from build123d import *

# Parameters (mm, degrees)
SKETCH1_W                   = 127
SKETCH1_H                   = 127
BOSS_EXTRUDE1_DEPTH         = 3.175
F_16_0_177_DIAMETER_HOLE1_D = 4.4958
F_16_0_177_DIAMETER_HOLE2_D = 4.4958
SKETCH12_W                  = 6.35
SKETCH12_H                  = 19.05
CUT_EXTRUDE1_DEPTH          = 131.218638569
FILLET1_R                   = 2.54


with BuildPart() as part:
    # Sketch1 → Boss-Extrude1 (new body)
    with BuildSketch(Plane(origin=(0, 0, 0), x_dir=(1, 0, 0), z_dir=(0, 1, 0))):
        with Locations((-41.826357018, 13.006024096)):
            Rectangle(SKETCH1_W, SKETCH1_H)
    extrude(amount=BOSS_EXTRUDE1_DEPTH)

    # #16 (0.177) Diameter Hole1 (through all)
    with Locations(Plane(origin=(0, 0, 0), x_dir=(-1, 0, 0), z_dir=(0, -1, 0))):
        with Locations((3.726357018, 63.806024096), (79.926357018, -37.793975904), (79.926357018, 63.806024096), (3.726357018, -37.793975904)):
            Hole(F_16_0_177_DIAMETER_HOLE1_D / 2)

    # #16 (0.177) Diameter Hole2 (through all)
    with Locations(Plane(origin=(0, 0, 0), x_dir=(-1, 0, 0), z_dir=(0, -1, 0))):
        with Locations((-10.624642982, 63.869524096), (94.277357018, -37.857475904), (94.277357018, 63.869524096), (-10.624642982, -37.857475904)):
            Hole(F_16_0_177_DIAMETER_HOLE2_D / 2)

    # Sketch12 → Cut-Extrude1 (cut, through all)
    with BuildSketch(Plane(origin=(0, 3.175, 0), x_dir=(1, 0, 0), z_dir=(0, 1, 0))):
        with Locations((18.498642982, -40.968975904)):
            Rectangle(SKETCH12_W, SKETCH12_H)
    extrude(amount=-CUT_EXTRUDE1_DEPTH, mode=Mode.SUBTRACT)

    # Fillet1
    fillet1_edges = [part.edges().sort_by_distance(p)[0] for p in [
        (15.323642982, 1.5875, 50.493975904),
        (15.323642982, 1.5875, 31.443975904),
        (21.673642982, 1.5875, 31.443975904),
        (-105.326357018, 1.5875, 50.493975904),
        (-105.326357018, 1.5875, -76.506024096),
        (21.673642982, 1.5875, -76.506024096),
    ]]
    fillet(fillet1_edges, radius=FILLET1_R)


solid = part.part
The listing builds one solid part. Answer for the finished solid, in the listing's coordinates (mm). Round coordinates to 2 decimals unless told otherwise and drop trailing zeros. Answer in a Markdown table with one row per item. Add a question column.
1) Determine the mould class of faces 1 (the face through (10.33, 1.61, -66.1)), 2 (the face through (15.324, 2, 41)), 3 (the face through (-43, 3.175, -14)) for opening direction X: pulls with the +X half, pulls with the -X half, needs draft (parallel to the pull), parting line crosses it, or undercut.
2) The part is cut by section A-A on y = 2.35. Count the separate pieces of the cut face and the enclosed holes in it, plus the area to 3 significant figures.
3) Consider line 1 along Z through (x, y) = (11.5, 1.25); line 2 along Z through (x, y) = (-95.5, 2.55); line 3 along Z through (x, y) = (14, 2.3). Determine where each line is inside the solid, lowest interval first. Write a range as from..to.
4) A flat-ended cylindrical pin translates along its axis: pin 1 Ø1 at (x, y) = (18.5, 1) entering from +Z. Find the tip coordinate at first contact, or state that the pin passes through.
Findings below:
| question | item | result |
|---|---|---|
| 1 | face 1 | undercut |
| 1 | face 2 | pulls with the +X half |
| 1 | face 3 | needs draft |
| 2 | separate pieces | 1 |
| 2 | enclosed holes | 8 |
| 2 | area | 15,900 mm² |
| 3 | line 1 | z = -76.51..-65.94, -61.8..35.79, 39.93..50.49 |
| 3 | line 2 | z = -76.51..-65.76, -61.98..35.97, 39.74..50.49 |
| 3 | line 3 | z = -76.51..50.18 |
| 4 | pin 1 | stops at z = 31.44 |
